The model under review builds one solid part; all positions refer to its coordinate system, in mm. Give positions to 0.01 mm unless a question says otherwise; leave off trailing zeros. Write each loop counter-clockwise with the first axis right and the second up, starting at its lowest first coordinate (ties: lowest second). Pieces come first, ordered by that corner, then holes. Notation, with made-up numbers: (68.5, 41.25) - (90.5, 41.25) arc R30 ccw to (90.5, 74.25) - close; hole circle Ø3 at (53.25, -3). An arc over 180 degrees is marked (long way). Write item = value, one per line.
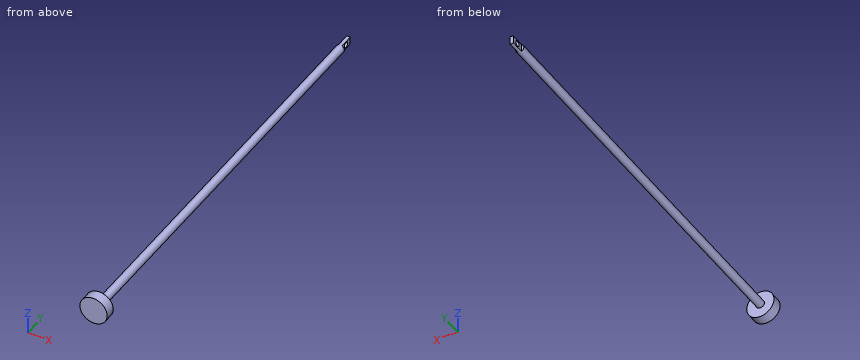
```python
from build123d import *

# Parameters (mm, degrees)
SKETCH_1_R           = 20
EXTRUDE_1_DEPTH      = 15
SKETCH_2_R           = 6
EXTRUDE_2_DEPTH      = 610
SKETCH_3_OUTSIDE_W   = 167.51
SKETCH_3_OUTSIDE_H   = 167.51
SKETCH_3_OUTSIDE_W_2 = 5
SKETCH_3_OUTSIDE_H_2 = 20
CUT_EXTRUDE_1_DEPTH  = 20
SKETCH_4_R           = 4
CUT_EXTRUDE_2_DEPTH  = 20


with BuildPart() as part:
    # 草图1 → 凸台-拉伸1 (new body)
    with BuildSketch(Plane(origin=(0, 0, 0), x_dir=(1, 0, 0), z_dir=(0, 1, 0))):
        Circle(SKETCH_1_R)
    extrude(amount=EXTRUDE_1_DEPTH)

    # 草图2 → 凸台-拉伸2 (add)
    with BuildSketch(Plane(origin=(0, 15, 0), x_dir=(1, 0, 0), z_dir=(0, 1, 0))):
        Circle(SKETCH_2_R)
    extrude(amount=EXTRUDE_2_DEPTH)

    # 草图3 outside → 切除-拉伸1 (cut)
    with BuildSketch(Plane(origin=(0, 625, 0), x_dir=(1, 0, 0), z_dir=(0, 1, 0))):
        Rectangle(SKETCH_3_OUTSIDE_W, SKETCH_3_OUTSIDE_H)
        Rectangle(SKETCH_3_OUTSIDE_W_2, SKETCH_3_OUTSIDE_H_2, mode=Mode.SUBTRACT)
    extrude(amount=-CUT_EXTRUDE_1_DEPTH, mode=Mode.SUBTRACT)

    # 草图4 → 切除-拉伸2 (cut)
    with BuildSketch(Plane.ZY.offset(2.5)):
        with Locations((0, 615)):
            Circle(SKETCH_4_R)
    extrude(amount=-CUT_EXTRUDE_2_DEPTH, mode=Mode.SUBTRACT)


solid = part.part
```
1. Take a section at B-B on y = 326.5. Give the boundary of the cut face in (x, z), and give its area (3 significant figures).
Findings below:
outline = circle Ø12 at (0, 0)
area = 113 mm²
2. Take a section at A-A on z = 12. Give the boundary of the cut face in (x, y), and give its area (3 significant figures).
Findings below:
outline = (-16, 0) - (16, 0) - (16, 15) - (-16, 15) - close
area = 480 mm²
3. For line 1 (Y direction, x = 1.1, z = 0); line 2 (Z direction, x = 1, y = 615); line 3 (Z direction, x = -0.15, y = 615), list the stretches that pass through material, from the lowest coordinate up. Write a range as from..to.
Findings below:
line_1 = 0..611, 619..625
line_2 = -5.92..-4, 4..5.92
line_3 = -6..-4, 4..6
4. Take a section at C-C on x = 11.5. Give the boundary of the cut face in (y, z).
Findings below:
outline = (0, -16.36) - (15, -16.36) - (15, 16.36) - (0, 16.36) - close
5. Insertion check: P1, Ø1.1, axis at x = 4.5, z = -1.5, coming from the +Y side; P2, Ø12, axis at x = 10, y = 457.5, coming from the +Z side; P3, Ø1.5, axis at x = -1.5, z = -9.5, coming from the +Y side. Each pin has a flat end and moves straight along its axis. Give the tip position at first contact, or say it passes through.
Findings below:
P1 = 605
P2 = 4.47
P3 = 15
